from build123d import *

# Parameters (mm, degrees)
SKETCH1_R           = 2
SKETCH1_R_2         = 11
SKETCH1_R_3         = 1.905
SKETCH1_R_4         = 2.5
SKETCH1_W           = 21.082
SKETCH1_H           = 40.64
BOSS_EXTRUDE1_DEPTH = 3.175
FILLET1_R           = 7.5


with BuildPart() as part:
    # Sketch1 → Boss-Extrude1 (new, symmetric)
    with BuildSketch(Plane.XY):
        Polygon((-20, -84), (20, -84), (20, 11), (35.179, 11), (35.179, 66), (-35.179, 66), (-35.179, 11), (-20, 11), align=None)
        with Locations((9.906, 11.938)):
            Circle(SKETCH1_R, mode=Mode.SUBTRACT)
        with Locations((-9.906, 11.938)):
            Circle(SKETCH1_R, mode=Mode.SUBTRACT)
        with Locations((-9.906, -11.938)):
            Circle(SKETCH1_R, mode=Mode.SUBTRACT)
        with Locations((9.906, -11.938)):
            Circle(SKETCH1_R, mode=Mode.SUBTRACT)
        with Locations((0, 38.5)):
            Circle(SKETCH1_R_2, mode=Mode.SUBTRACT)
        with Locations((15.494, 53.994)):
            Circle(SKETCH1_R_3, mode=Mode.SUBTRACT)
        with Locations((-5.1689, -30)):
            Circle(SKETCH1_R, mode=Mode.SUBTRACT)
        with Locations((5.2451, -30)):
            Circle(SKETCH1_R, mode=Mode.SUBTRACT)
        with Locations((5.2451, -79.784)):
            Circle(SKETCH1_R, mode=Mode.SUBTRACT)
        with Locations((-5.1689, -79.784)):
            Circle(SKETCH1_R, mode=Mode.SUBTRACT)
        with Locations((-26.67, 38.5)):
            Circle(SKETCH1_R_4, mode=Mode.SUBTRACT)
        with Locations((26.67, 38.5)):
            Circle(SKETCH1_R_4, mode=Mode.SUBTRACT)
        with Locations((15.494, 23.006)):
            Circle(SKETCH1_R_3, mode=Mode.SUBTRACT)
        with Locations((-15.494, 23.006)):
            Circle(SKETCH1_R_3, mode=Mode.SUBTRACT)
        with Locations((-15.494, 53.994)):
            Circle(SKETCH1_R_3, mode=Mode.SUBTRACT)
        with BuildLine():
            Line((8.804893639, 49.100944864), (11.319365353, 51.615416577))
            ThreePointArc((11.319365353, 51.615416577), (13.115416577, 51.615416577), (13.115416577, 49.819365353))
            Line((13.115416577, 49.819365353), (10.600944864, 47.304893639))
            ThreePointArc((10.600944864, 47.304893639), (8.804893639, 47.304893639), (8.804893639, 49.100944864))
        make_face(mode=Mode.SUBTRACT)
        with Locations((0, -54.892)):
            Rectangle(SKETCH1_W, SKETCH1_H, mode=Mode.SUBTRACT)
        with BuildLine():
            Line((10.600944864, 29.695106361), (13.115416577, 27.180634647))
            ThreePointArc((13.115416577, 27.180634647), (13.115416577, 25.384583423), (11.319365353, 25.384583423))
            Line((11.319365353, 25.384583423), (8.804893639, 27.899055136))
            ThreePointArc((8.804893639, 27.899055136), (8.804893639, 29.695106361), (10.600944864, 29.695106361))
        make_face(mode=Mode.SUBTRACT)
        with BuildLine():
            Line((-8.804893639, 27.899055136), (-11.319365353, 25.384583423))
            ThreePointArc((-11.319365353, 25.384583423), (-13.115416577, 25.384583423), (-13.115416577, 27.180634647))
            Line((-13.115416577, 27.180634647), (-10.600944864, 29.695106361))
            ThreePointArc((-10.600944864, 29.695106361), (-8.804893639, 29.695106361), (-8.804893639, 27.899055136))
        make_face(mode=Mode.SUBTRACT)
        with BuildLine():
            Line((-10.600944864, 47.304893639), (-13.115416577, 49.819365353))
            ThreePointArc((-13.115416577, 49.819365353), (-13.115416577, 51.615416577), (-11.319365353, 51.615416577))
            Line((-11.319365353, 51.615416577), (-8.804893639, 49.100944864))
            ThreePointArc((-8.804893639, 49.100944864), (-8.804893639, 47.304893639), (-10.600944864, 47.304893639))
        make_face(mode=Mode.SUBTRACT)
    extrude(amount=BOSS_EXTRUDE1_DEPTH, both=True)

    # Fillet1
    fillet1_edges = [part.edges().sort_by_distance(p)[0] for p in [
        (20, -84, 0),
        (-20, -84, 0),
        (-20, 11, 0),
        (-35.179, 11, 0),
        (-35.179, 66, 0),
        (35.179, 66, 0),
        (35.179, 11, 0),
        (20, 11, 0),
    ]]
    fillet(fillet1_edges, radius=FILLET1_R)


solid = part.part
Verification items for the finished model (mm, model axes). A direction names the side the tool comes from. Coordinates: 2 decimals unless noted, no trailing zeros. Order: outer loops, then holes, each group sorted by start corner. A loop starts at its lowest first (then second) coordinate and runs counter-clockwise, first axis right, second up. Notation, with made-up numbers: M 53,81 L 95,81 A15 ccw 95,97 Z; hole C 10.5,-13 d4. An arc over 180 degrees is marked long. Return JSON: item names as keys, results as strings.
1) Cross-section at D-D, the plane y = -61.5. Record the boundary of the cut face in (x, z) (3 decimals), and give its area (3 significant figures).
Answer list:
{"outline": "M -20,-3.175 L -10.541,-3.175 L -10.541,3.175 L -20,3.175 Z; M 10.541,-3.175 L 20,-3.175 L 20,3.175 L 10.541,3.175 Z", "area": "120 mm2"}
2) Access from +Z, -Z, +X, -X, +Y, -Y to the whole of each face (thin tool, end or side, straight path). Record for faces 1 (the flat face through (-20, -36, 0)), 2 (the flat face through (0, -75.212, 0)), 3 (the flat face through (0, 9, 3.175)).
Answer list:
{"face 1": "+Z, -Z, -X, -Y", "face 2": "+Z, -Z", "face 3": "+Z, +X, -X, +Y, -Y"}
3) Thickness scan on L1, parallel to Y at x = 3, z = -0.25; L2, parallel to X at y = -43.5, z = -2.5; L3, parallel to Y at x = 6.5, z = -0.75. Record the ranges inside material, lowest first. Write a range as [from, to].
Answer list:
{"L1": "[-84, -75.21], [-34.57, 27.92], [49.08, 66]", "L2": "[-20, -10.54], [10.54, 20]", "L3": "[-84, -81.34], [-78.23, -75.21], [-34.57, -31.56], [-28.44, 29.63], [47.37, 66]"}
4) Cross-section at B-B, the plane y = 38.5. Record the boundary of the cut face in (x, z) (3 decimals), and give its area (3 significant figures).
Answer list:
{"outline": "M -35.179,-3.175 L -29.17,-3.175 L -29.17,3.175 L -35.179,3.175 Z; M -24.17,-3.175 L -11,-3.175 L -11,3.175 L -24.17,3.175 Z; M 11,-3.175 L 24.17,-3.175 L 24.17,3.175 L 11,3.175 Z; M 29.17,-3.175 L 35.179,-3.175 L 35.179,3.175 L 29.17,3.175 Z", "area": "244 mm2"}
5) Cross-section at A-A, the plane y = -30. Record the boundary of the cut face in (x, z) (3 decimals), and give its area (3 significant figures).
Answer list:
{"outline": "M -20,-3.175 L -7.169,-3.175 L -7.169,3.175 L -20,3.175 Z; M -3.169,-3.175 L 3.245,-3.175 L 3.245,3.175 L -3.169,3.175 Z; M 7.245,-3.175 L 20,-3.175 L 20,3.175 L 7.245,3.175 Z", "area": "203 mm2"}
6) Release check for a two-part mould opening along Y. For faces 4 (the cylindrical face through (-22.139, 8.745, -0.044)), 5 (the flat face through (10.08, 26.624, 0.044)), 6 (the flat face through (20, -37, 0)) record: +Y half, -Y half, draft (parallel to the pull), parting line (faces both ways), or undercut.
Answer list:
{"face 4": "-Y half", "face 5": "undercut", "face 6": "draft"}
7) Cross-section at C-C, the plane x = -26. Record the boundary of the cut face in (y, z) (3 decimals).
Answer list:
{"outline": "M 10.848,-3.175 L 36.091,-3.175 L 36.091,3.175 L 10.848,3.175 Z; M 40.909,-3.175 L 66,-3.175 L 66,3.175 L 40.909,3.175 Z"}
8) Gauge pin test, flat end, axial feed: pin 1 (3 mm diameter, centred on y = 6, z = 1.5, fed in from +X). Record the tip position at first contact, or that the pin passes through.
Answer list:
{"pin 1": "x = 21.16"}
